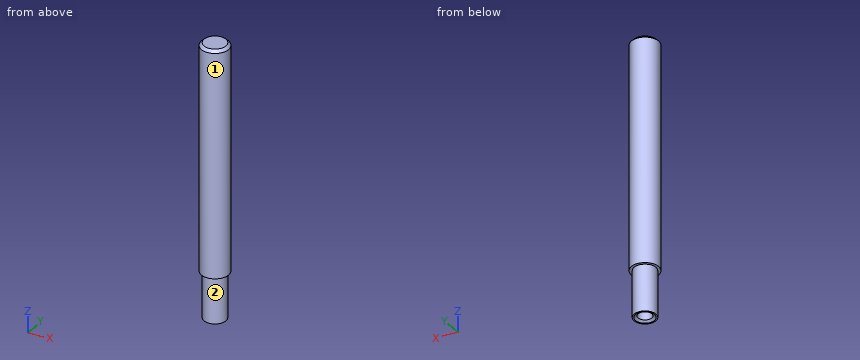
from build123d import *

# Parameters (mm, degrees)
ESQUISSE1_R                 = 4
BOSS_EXTRU_1_DEPTH          = 17
ESQUISSE2_R                 = 5
BOSS_EXTRU_2_DEPTH          = 83
CHANFREIN1_SIZE             = 1
TROU_TARAUD_M61_D           = 5
TROU_TARAUD_M61_DEPTH       = 15
TROU_TARAUD_M61_CSINK_D     = 7
TROU_TARAUD_M61_CSINK_ANGLE = 120
TROU_TARAUD_M61_TIP         = 1.502151548


with BuildPart() as part:
    # Esquisse1 → Boss.-Extru.1 (new body)
    with BuildSketch(Plane.XY):
        Circle(ESQUISSE1_R)
    extrude(amount=BOSS_EXTRU_1_DEPTH)

    # Esquisse2 → Boss.-Extru.2 (add)
    with BuildSketch(Plane.XY.offset(17)):
        Circle(ESQUISSE2_R)
    extrude(amount=BOSS_EXTRU_2_DEPTH)

    # Chanfrein1
    chanfrein1_edges = [part.edges().sort_by_distance(p)[0] for p in [
        (-5, 0, 100),
    ]]
    chamfer(chanfrein1_edges, length=CHANFREIN1_SIZE)

    # Trou taraudé M61
    with Locations(Plane(origin=(0, 0, 0), x_dir=(-1, 0, 0), z_dir=(0, 0, -1))):
        with Locations((0, 0)):
            CounterSinkHole(TROU_TARAUD_M61_D / 2, TROU_TARAUD_M61_CSINK_D / 2, depth=TROU_TARAUD_M61_DEPTH, counter_sink_angle=TROU_TARAUD_M61_CSINK_ANGLE)
            with Locations((0, 0, -(TROU_TARAUD_M61_DEPTH + TROU_TARAUD_M61_TIP / 2))):  # 118° drill point
                Cone(0, TROU_TARAUD_M61_D / 2, TROU_TARAUD_M61_TIP, mode=Mode.SUBTRACT)


solid = part.part
Work out the finished part from the listing and answer in its coordinate system (mm). Face numbers are marked on the shaded views. A direction names the side the tool comes from. Round coordinates to 2 decimals unless told otherwise and drop trailing zeros. Order: outer loops, then holes, each group sorted by start corner. A loop starts at its lowest first (then second) coordinate and runs counter-clockwise, first axis right, second up. Notation, with made-up numbers: M -29.5,-28 L 24.5,-28 A25 cw 24.5,-8 Z; hole C -13.5,7 d8. An arc over 180 degrees is marked long. Put each result on its own line as item: value. Start each with the question number.
Q1. Straight lines are drawn through the part: L1, parallel to Y at x = 0, z = 4.75; L2, parallel to Y at x = 3, z = 19; L3, parallel to X at y = -3.5, z = 62. For each, find the intervals that lie inside material, in ascending order. Write a range as [from, to].
Q2. Section A-A, the plane z = 91.5 is taken. Write down the section's boundary in (x, y).
Q3. Flat-ended cylindrical pins translate along their axes: pin 1 (2 mm diameter, centred on y = -2.5, z = 24, fed in from +X); pin 2 (3 mm diameter, centred on y = -3, z = 17.5, fed in from -X); pin 3 (1 mm diameter, centred on x = -1, z = 38.5, fed in from +Y). Find the tip coordinate at first contact, or state that the pin passes through.
Q4. A tool of negligible diameter and unlimited length cuts with its end or side. For the marked faces 1 and 2, from which of +Z, -Z, +X, -X, +Y, -Y can it reach the whole face along a straight path? Write none if from no direction.
Findings below:
1. L1: y = [-4, -2.5], [2.5, 4]
1. L2: y = [-4, 4]
1. L3: x = [-3.57, 3.57]
2. outline: C 0,0 d10
3. pin 1: stops at x = 4.77
3. pin 2: stops at x = -4.77
3. pin 3: stops at y = 4.97
4. face 1: +Z, -Z
4. face 2: -Z
